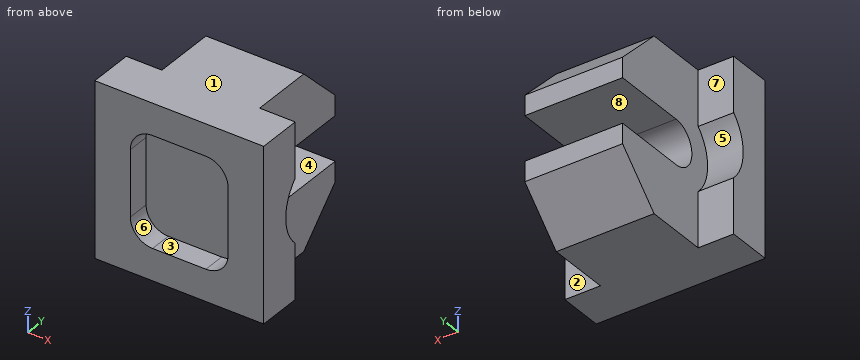
Autodesk Inventor part; units mm, degrees
ref_plane "Work Plane1" through (0, 0, 0) normal (1, 0, 0) x (0, 1, 0)
ref_plane "XZ Plane" through (0, 0, 0) normal (0, 1, 0) x (-1, 0, 0)
ref_plane "XY Plane" through (0, 0, 0) normal (0, 0, 1) x (1, 0, 0)
sketch "Sketch1" plane through (0, 0, 0) normal (0, 1, 0) x (-1, 0, 0)
  line L0 (9.5, 9.75) -> (-9.5, 9.75)
  line L1 (-9.5, 9.75) -> (-9.5, -9.75)
  line L2 (-9.5, -9.75) -> (9.5, -9.75)
  line L3 (9.5, -9.75) -> (9.5, 9.75)
  line L4 (9.5, 9.75) -> (-9.5, -9.75) construction
  line L5 (-9.5, 9.75) -> (9.5, -9.75) construction
  point P0 (0, 0)
  dimension "d0" = 19
  dimension "d1" = 19.5
extrude "Extrusion1" add sketch "Sketch1" along normal blind 5
sketch "Sketch2" plane through (0, 0, 0) normal (0, -1, 0) x (1, 0, 0)
  line L0 (5.5, 6.2) -> (-5.5, 6.2)
  line L1 (-5.5, 6.2) -> (-5.5, -6.2)
  line L2 (-5.5, -6.2) -> (5.5, -6.2)
  line L3 (5.5, -6.2) -> (5.5, 6.2)
  line L4 (5.5, 6.2) -> (-5.5, -6.2) construction
  line L5 (-5.5, 6.2) -> (5.5, -6.2) construction
  point P0 (0, 0)
  dimension "d4" = 11
  dimension "d5" = 12.4
extrude "Extrusion2" cut sketch "Sketch2" against normal blind 2.5
fillet "Fillet1" radius 2.5 4 edges at (-5.5, 1.25, 6.2) (5.5, 1.25, 6.2) (5.5, 1.25, -6.2) (-5.5, 1.25, -6.2)
sketch "Sketch3" plane through (0, 5, 0) normal (0, 1, 0) x (1, 0, 0)
  line L0 (9.5, 9.75) -> (-9.5, 9.75)
  line L1 (-5.5, -9.75) -> (5.5, -9.75)
  line L2 (5.5, -9.75) -> (5.5, 9.75)
  line L3 (5.5, 9.75) -> (-5.5, 9.75)
  line L4 (-5.5, 9.75) -> (-5.5, -9.75)
  line L5 (-5.5, -9.75) -> (5.5, 9.75) construction
  line L6 (5.5, -9.75) -> (-5.5, 9.75) construction
  point P0 (0, 0)
  dimension "d9" = 11
extrude "Extrusion3" add sketch "Sketch3" along normal blind 12
chamfer "Chamfer1" distance 5 angle 45 2 edges at (0, 17, 9.75) (0, 17, -9.75)
sketch "Sketch4" plane through (5.5, 5, 9.75) normal (1, 0, 0) x (0, 0, -1)
  line L0 (12.25, 20.5) -> (7.25, 20.5)
  line L1 (7.25, 20.5) -> (7.25, 3.5)
  line L2 (7.25, 3.5) -> (12.25, 3.5)
  line L3 (12.25, 3.5) -> (12.25, 20.5)
  line L4 (14.5, 12) -> (5, 12)
  line L5 (12.25, 20.5) -> (7.25, 3.5) construction
  line L6 (7.25, 20.5) -> (12.25, 3.5) construction
  circle A0 centre (9.75, 3.5) radius 2.5
  point P0 (9.75, -5)
  point P1 (9.75, 12)
  dimension "d15" = 5
  dimension "d16" = 17
extrude "Extrusion4" cut sketch "Sketch4" against normal through all
sketch "Sketch5" plane through (9.5, 0, 9.75) normal (1, 0, 0) x (0, 0, -1)
  arc A0 (7.25, 8.5) -> (12.25, 8.5) centre (9.75, 8.5) ccw
  circle A1 centre (9.75, 8.5) radius 5
  point P0 (9.75, 0)
  dimension "d19" = 10
extrude "Extrusion5" cut sketch "Sketch5" against normal up to surface (4 mm away)
ref_plane "Work Plane1" through (0, 0, 0) normal (1, 0, 0) x (0, 1, 0)
mirror "Mirror1" about plane through (0, 0, 0) normal (1, 0, 0) of "Extrusion5"
properties part number "Cassetto"
Geometry check sheet. Reference: the model listing, model coordinates, mm. Face numbers are marked on the shaded views. A direction names the side the tool comes from. Coordinates: 2 decimals unless noted, no trailing zeros. Write each loop counter-clockwise with the first axis right and the second up, starting at its lowest first coordinate (ties: lowest second). Pieces come first, ordered by that corner, then holes. Notation, with made-up numbers: M 63.5,42.5 L 81.5,42.5 A12 cw 81.5,51.5 Z; hole C 49,17 d4. An arc over 180 degrees is marked long. Use one line per item in the form item = value. Start each with the question number.
1) Section check B-B on z = 0. Enter the section's corners in (x, y).
2) Release check for a two-part mould opening along Z. For the marked faces 1, 2, 3 and 4 record: pulls with the +Z half, pulls with the -Z half, needs draft (parallel to the pull), parting line crosses it, or undercut.
3) Section check C-C on x = -4.5. Enter the section's corners in (y, z), and give its area (3 significant figures).
4) Section check A-A on y = 16. Enter the section's corners in (x, z), and give its area (3 significant figures).
5) Go/stop test with flat-tipped pins: pin 1 Ø7 at (y, z) = (10.5, 0) entering from +X; pin 2 Ø4.5 at (x, z) = (-7.5, -6) entering from +Y; pin 3 Ø1.2 at (x, z) = (-7, 7) entering from +Y. Record where each tip stops, or that it passes through.
6) Section check D-D on y = 13. Enter the section's corners in (x, z).
7) Thickness scan on probe 1 along Z at (x, y) = (-0.5, 10); probe 2 along X at (y, z) = (6, 6); probe 3 along Y at (x, z) = (8.25, -0.25). Record the ranges inside material, lowest first. Write a range as from..to.
8) Set-up check for the marked faces 5, 6, 7 and 8: record each of +Z, -Z, +X, -X, +Y, -Y from which the full face is reachable in a straight line by a thin tool's end or side.
Responses:
q1.outline = M -9.5,0 L -5.5,0 L -5.5,2.5 L 5.5,2.5 L 5.5,0 L 9.5,0 L 9.5,3.5 L 5.5,3.5 L 5.5,6 L -5.5,6 L -5.5,3.5 L -9.5,3.5 Z
q2.face_1 = pulls with the +Z half
q2.face_2 = needs draft
q2.face_3 = undercut
q2.face_4 = undercut
q3.outline = M 0,-9.75 L 12,-9.75 L 17,-4.75 L 17,-2.5 L 8.5,-2.5 A2.5 cw 8.5,2.5 L 17,2.5 L 17,4.75 L 12,9.75 L 0,9.75 L 0,5.7 L 2.5,5.7 L 2.5,-5.7 L 0,-5.7 Z
q3.area = 226 mm2
q4.outline = M -5.5,-5.75 L 5.5,-5.75 L 5.5,-2.5 L -5.5,-2.5 Z; M -5.5,2.5 L 5.5,2.5 L 5.5,5.75 L -5.5,5.75 Z
q4.area = 71.5 mm2
q5.pin_1 = 5.5
q5.pin_2 = 16.78
q5.pin_3 = 5
q6.outline = M -5.5,-8.75 L 5.5,-8.75 L 5.5,-2.5 L -5.5,-2.5 Z; M -5.5,2.5 L 5.5,2.5 L 5.5,8.75 L -5.5,8.75 Z
q7.probe_1 = -9.75..-2.5, 2.5..9.75
q7.probe_2 = -5.5..5.5
q7.probe_3 = 0..3.51
q8.face_5 = -X, +Y
q8.face_6 = -Y
q8.face_7 = +Z, -Z, -X, +Y
q8.face_8 = +X, -X, +Y
